Drawing for the job (mm, zero at the part's lowest x, y, z). A direction names the side the tool comes from. Round coordinates to 2 decimals unless told otherwise and drop trailing zeros. Loops run counter-clockwise (first coordinate to the right, second up) from the corner with the lowest first, then second, coordinate; pieces in that order, holes last. Notation, with made-up numbers: (-37, 2.5) - (-17, 2.5) arc R11 ccw to (-17, 10.5) - close; hole circle Ø11 at (25, -0.75). An arc over 180 degrees is marked (long way). Put each result on its own line as item: value.
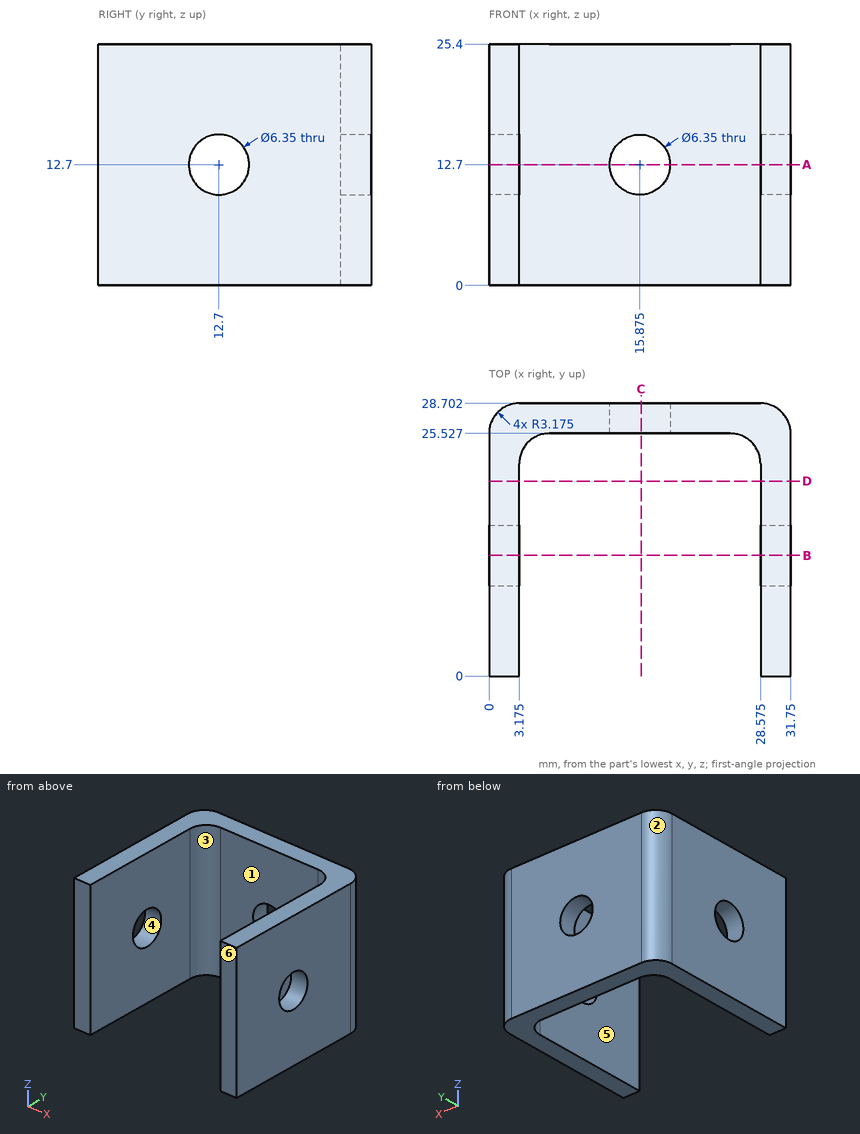
1. Probe line 1 along X through (y, z) = (2, 13.75) (3 decimals); line 2 along Y through (x, z) = (25.5, 18); line 3 along X through (y, z) = (23.75, 11.25). List the from-to ranges inside material, lowest first. Write a range as [from, to].
A:
line 1: x = [0, 3.175], [28.575, 31.75]
line 2: y = [25.53, 28.7]
line 3: x = [0, 3.5], [28.25, 31.75]
2. Tool access for the marked faces 5 and 6: list every direction of +Z, -Z, +X, -X, +Y, -Y with a clear straight run to the whole face (end or side of a thin tool).
A:
face 5: +Z, -Z, -Y
face 6: +Z, -Z, +X, -X, -Y
3. Band-saw the part on C-C (x = 16). List the corners of the cut face in (y, z).
A:
outline: (25.53, 0) - (28.7, 0) - (28.7, 9.53) - (25.53, 9.53) - close; (25.53, 15.87) - (28.7, 15.87) - (28.7, 25.4) - (25.53, 25.4) - close
4. Band-saw the part on B-B (y = 12.7). List the corners of the cut face in (x, z) (3 decimals).
A:
outline: (0, 0) - (3.175, 0) - (3.175, 9.525) - (0, 9.525) - close; (0, 15.875) - (3.175, 15.875) - (3.175, 25.4) - (0, 25.4) - close; (28.575, 0) - (31.75, 0) - (31.75, 9.525) - (28.575, 9.525) - close; (28.575, 15.875) - (31.75, 15.875) - (31.75, 25.4) - (28.575, 25.4) - close
5. Band-saw the part on A-A (z = 12.7). List the corners of the cut face in (x, y) (3 decimals), plus the area to 3 significant figures.
A:
outline: (0, 0) - (3.175, 0) - (3.175, 9.525) - (0, 9.525) - close; (0, 15.875) - (3.175, 15.875) - (3.175, 22.352) arc R3.175 cw to (6.35, 25.527) - (12.7, 25.527) - (12.7, 28.702) - (3.175, 28.702) arc R3.175 ccw to (0, 25.527) - close; (19.05, 25.527) - (25.4, 25.527) arc R3.175 cw to (28.575, 22.352) - (28.575, 15.875) - (31.75, 15.875) - (31.75, 25.527) arc R3.175 ccw to (28.575, 28.702) - (19.05, 28.702) - close; (28.575, 0) - (31.75, 0) - (31.75, 9.525) - (28.575, 9.525) - close
area: 202 mm²
6. Pin check, flat tips, straight feed: P1, Ø5, axis at x = 25, y = 8.5, coming from the +Z side; P2, Ø9.5, axis at x = 14, z = 17.5, coming from the -Y side. Stop position of each tip, or through.
A:
P1: passes through
P2: stops at y = 25.53
7. Two-plate mould, pull along X, no slides. Class the marked faces 1, 2, 3 and 4: pulls with the +X half, pulls with the -X half, needs draft (parallel to the pull), parting line crosses it, or undercut.
A:
face 1: undercut
face 2: pulls with the -X half
face 3: undercut
face 4: needs draft
8. Band-saw the part on D-D (y = 20.5). List the corners of the cut face in (x, z) (3 decimals).
A:
outline: (0, 0) - (3.175, 0) - (3.175, 25.4) - (0, 25.4) - close; (28.575, 0) - (31.75, 0) - (31.75, 25.4) - (28.575, 25.4) - close
